from build123d import *

# Parameters (mm, degrees)
SKETCH_W      = 19
SKETCH_H      = 52
SKETCH_R      = 2.6
SKETCH_W_2    = 9
SKETCH_H_2    = 14
PAD_DEPTH     = 3
SKETCH001_W   = 19
SKETCH001_H   = 24
SKETCH001_W_2 = 9
SKETCH001_H_2 = 14
PAD001_DEPTH  = 17
FILLET_R      = 5
FILLET001_R   = 3
FILLET002_R   = 3
FILLET003_R   = 3
SKETCH002_W   = 5
SKETCH002_H   = 3
POCKET_DEPTH  = 5


with BuildPart() as part:
    # Sketch → Pad (new body)
    with BuildSketch(Plane.XY):
        with Locations((4.5, 7)):
            Rectangle(SKETCH_W, SKETCH_H)
        with Locations((4.5, -13)):
            Circle(SKETCH_R, mode=Mode.SUBTRACT)
        with Locations((4.5, 27)):
            Circle(SKETCH_R, mode=Mode.SUBTRACT)
        with Locations((4.5, 7)):
            Rectangle(SKETCH_W_2, SKETCH_H_2, mode=Mode.SUBTRACT)
    extrude(amount=PAD_DEPTH)

    # Sketch001 → Pad001 (join)
    with BuildSketch(Plane.XY):
        with Locations((4.5, 7)):
            Rectangle(SKETCH001_W, SKETCH001_H)
        with Locations((4.5, 7)):
            Rectangle(SKETCH001_W_2, SKETCH001_H_2, mode=Mode.SUBTRACT)
    extrude(amount=PAD001_DEPTH)

    # Fillet
    fillet_edges = [part.edges().sort_by_distance(p)[0] for p in [
        (14, -19, 1.5),
        (-5, -19, 1.5),
        (14, 33, 1.5),
        (-5, 33, 1.5),
    ]]
    fillet(fillet_edges, radius=FILLET_R)

    # Fillet001
    fillet001_edges = [part.edges().sort_by_distance(p)[0] for p in [
        (14, -5, 10),
    ]]
    fillet(fillet001_edges, radius=FILLET001_R)

    # Fillet002
    fillet002_edges = [part.edges().sort_by_distance(p)[0] for p in [
        (-5, -5, 10),
        (-5, 19, 10),
    ]]
    fillet(fillet002_edges, radius=FILLET002_R)

    # Fillet003
    fillet003_edges = [part.edges().sort_by_distance(p)[0] for p in [
        (14, 19, 10),
    ]]
    fillet(fillet003_edges, radius=FILLET003_R)

    # Sketch002 (on Face16 of Fillet003) → Pocket (cut)
    with BuildSketch(Plane(origin=(-5, 0, 0), x_dir=(0, -1, 0), z_dir=(-1, 0, 0))):
        with Locations((-2.5, 1.5)):
            Rectangle(SKETCH002_W, SKETCH002_H)
    extrude(amount=-POCKET_DEPTH, mode=Mode.SUBTRACT)


solid = part.part
The model under review builds one solid part; all positions refer to its coordinate system, in mm. A direction names the side the tool comes from. Round coordinates to 2 decimals unless told otherwise and drop trailing zeros. Loops run counter-clockwise (first coordinate to the right, second up) from the corner with the lowest first, then second, coordinate; pieces in that order, holes last. Notation, with made-up numbers: (-25.5, 23) -> (23.5, 23) arc R24 ccw to (23.5, 37) -> close; hole circle Ø1 at (-8.75, 60.5). An arc over 180 degrees is marked (long way). Answer as CSV lines item,"result".
1) Add section C-C on z = 6.5. Write out the cut boundary in (x, y).
Geometry results:
outline,"(-5, -2) arc R3 ccw to (-2, -5) -> (11, -5) arc R3 ccw to (14, -2) -> (14, 16) arc R3 ccw to (11, 19) -> (-2, 19) arc R3 ccw to (-5, 16) -> close; hole (0, 0) -> (9, 0) -> (9, 14) -> (0, 14) -> close"
2) For P1, Ø1.5, axis at x = -3, z = 1.5, coming from the -Y side; P2, Ø10, axis at x = 6.5, z = 10, coming from the -Y side; P3, Ø8.5, axis at x = 4.5, y = -13, coming from the +Z side; P4, Ø2, axis at y = 21.5, z = 6, coming from the -X side, all flat-tipped, find the tip position at first contact; note any pin that passes through.
Geometry results:
P1,"stops at y = -18.47"
P2,"stops at y = -5"
P3,"stops at z = 3"
P4,"passes through"
3) To check wall thickness, follow line 1 along Y through (x, z) = (4.5, 2); line 2 along Y through (x, z) = (7.5, 14.75); line 3 along X through (y, z) = (2.5, 14.25). State the ranges of each line that lie inside material, in increasing order. Write a range as from..to.
Geometry results:
line 1,"y = -19..-15.6, -10.4..0, 14..24.4, 29.6..33"
line 2,"y = -5..0, 14..19"
line 3,"x = -5..0, 9..14"
4) Draft analysis for pull direction Y (two halves, no side actions). For faces 4 (the face through (-4, 31, 2)), 5 (the face through (-3, 3, 3)), 6 (the face through (14, 7, 6)), state which applies: pulls with the +Y half, pulls with the -Y half, needs draft (parallel to the pull), parting line crosses it, or undercut.
Geometry results:
face 4,"pulls with the +Y half"
face 5,"undercut"
face 6,"needs draft"
5) Add section D-D on y = -13. Write out the cut boundary in (x, z).
Geometry results:
outline,"(-5, 0) -> (1.9, 0) -> (1.9, 3) -> (-5, 3) -> close; (7.1, 0) -> (14, 0) -> (14, 3) -> (7.1, 3) -> close"
6) Tool access review of faces 1 (the face through (4, -5, 10)), 2 (the face through (-4.1, 18.14, 10.1)), 3 (the face through (0, 7, 8)): name each direction out of +Z, -Z, +X, -X, +Y, -Y from which nothing blocks a thin tool from reaching the whole face with its end or side.
Geometry results:
face 1,"+Z, +X, -X, -Y"
face 2,"+Z, -X, +Y"
face 3,"+Z, -Z"
7) Add section B-B on y = 7. Write out the cut boundary in (x, z), plus the area to 3 significant figures.
Geometry results:
outline,"(-5, 0) -> (0, 0) -> (0, 17) -> (-5, 17) -> close; (9, 0) -> (14, 0) -> (14, 17) -> (9, 17) -> close"
area,"170 mm²"
8) Add section A-A on x = 4.5. Write out the cut boundary in (y, z).
Geometry results:
outline,"(-19, 0) -> (-15.6, 0) -> (-15.6, 3) -> (-19, 3) -> close; (-10.4, 0) -> (0, 0) -> (0, 17) -> (-5, 17) -> (-5, 3) -> (-10.4, 3) -> close; (14, 0) -> (24.4, 0) -> (24.4, 3) -> (19, 3) -> (19, 17) -> (14, 17) -> close; (29.6, 0) -> (33, 0) -> (33, 3) -> (29.6, 3) -> close"
